Geometry: final body of the model. Coordinates: model frame, mm. A direction names the side the tool comes from. Coordinates: 2 decimals unless noted, no trailing zeros. Write each loop counter-clockwise with the first axis right and the second up, starting at its lowest first coordinate (ties: lowest second). Pieces come first, ordered by that corner, then holes. Notation, with made-up numbers: (-24, 31) - (-18, 31) arc R27 cw to (-18, 52) - close; hole circle Ø4 at (71, 57). An arc over 180 degrees is marked (long way). Put each result on its own line as item: value.
```python
from build123d import *

# Parameters (mm, degrees)
SKETCH1_W           = 57.15
SKETCH1_H           = 50.8
BOSS_EXTRUDE1_DEPTH = 63.5
SKETCH2_R           = 9.506140486
CUT_EXTRUDE1_DEPTH  = 6.35
FILLET1_R           = 7.874
SKETCH3_W           = 47.524607072
SKETCH3_H           = 34.745914464
CUT_EXTRUDE2_DEPTH  = 57.15
FILLET2_R           = 3.81
SKETCH4_R           = 4.44219446
CUT_EXTRUDE3_DEPTH  = 5.08
CUT_EXTRUDE4_DEPTH  = 25.4


with BuildPart() as part:
    # Sketch1 → Boss-Extrude1 (new body)
    with BuildSketch(Plane.XY):
        with Locations((28.575, 25.4)):
            Rectangle(SKETCH1_W, SKETCH1_H)
    extrude(amount=BOSS_EXTRUDE1_DEPTH)

    # Sketch2 → Cut-Extrude1 (cut)
    with BuildSketch(Plane.XY.offset(63.5)):
        with Locations((25.4, 20.32)):
            Circle(SKETCH2_R)
    extrude(amount=-CUT_EXTRUDE1_DEPTH, mode=Mode.SUBTRACT)

    # Fillet1
    fillet1_edges = [part.edges().sort_by_distance(p)[0] for p in [
        (28.575, 50.8, 63.5),
    ]]
    fillet(fillet1_edges, radius=FILLET1_R)

    # Sketch3 → Cut-Extrude2 (cut)
    with BuildSketch(Plane(origin=(57.15, 0, 0), x_dir=(0, 0, -1), z_dir=(1, 0, 0))):
        with Locations((-23.762303536, 17.372957232)):
            Rectangle(SKETCH3_W, SKETCH3_H)
    extrude(amount=-CUT_EXTRUDE2_DEPTH, mode=Mode.SUBTRACT)

    # Fillet2
    fillet2_edges = [part.edges().sort_by_distance(p)[0] for p in [
        (28.575, 34.745914464, 47.524607072),
    ]]
    fillet(fillet2_edges, radius=FILLET2_R)

    # Sketch4 → Cut-Extrude3 (cut)
    with BuildSketch(Plane(origin=(57.15, 0, 0), x_dir=(0, 0, -1), z_dir=(1, 0, 0))):
        with Locations((-55.906607072, 43.18)):
            Circle(SKETCH4_R)
    extrude(amount=-CUT_EXTRUDE3_DEPTH, mode=Mode.SUBTRACT)

    # Sketch5 → Cut-Extrude4 (cut)
    with BuildSketch(Plane(origin=(0, 50.8, 0), x_dir=(1, 0, 0), z_dir=(0, 1, 0))):
        with BuildLine():
            Line((14.081947764, 0), (43.068052236, 0))
            ThreePointArc((43.068052236, 0), (28.575, -14.493052236), (14.081947764, 0))
        make_face()
    extrude(amount=-CUT_EXTRUDE4_DEPTH, mode=Mode.SUBTRACT)


solid = part.part
```
1. Section query A-A (y = 20.32). Return loops of the section in (x, z), then the cut area to 3 significant figures.
Answer below:
outline: (0, 47.52) - (57.15, 47.52) - (57.15, 63.5) - (34.91, 63.5) - (34.91, 57.15) - (15.89, 57.15) - (15.89, 63.5) - (0, 63.5) - close
area: 792 mm²
2. Ray query, probe 1 along Z at (x, y) = (53, 43); probe 2 along Z at (x, y) = (35.5, 8); probe 3 along Y at (x, z) = (25.4, 59.5). Return the intervals inside material, ascending. Write a range as from..to.
Answer below:
probe 1: z = 0..51.47, 60.35..63.5
probe 2: z = 47.52..63.5
probe 3: y = 0..10.81, 29.83..49.78
3. Set-up query: faces 5 (the flat face through (28, 50.8, 27)), 6 (the flat face through (52.07, 43, 56)), 7 (the flat face through (29, 34.746, 27)). Return all of +Z, -Z, +X, -X, +Y, -Y with unobstructed straight access to the full face (end or side cutting, diameter ignored); none if empty.
Answer below:
face 5: +Z, -Z, +X, -X, +Y
face 6: +X
face 7: -Z, +X, -X, -Y
4. Section query D-D (z = 27). Return loops of the section in (x, y), then the cut area to 3 significant figures.
Answer below:
outline: (0, 34.75) - (57.15, 34.75) - (57.15, 50.8) - (0, 50.8) - close
area: 917 mm²
5. Section query C-C (z = 59). Return loops of the section in (x, y), then the cut area to 3 significant figures.
Answer below:
outline: (0, 0) - (57.15, 0) - (57.15, 39.99) - (52.07, 39.99) - (52.07, 46.37) - (57.15, 46.37) - (57.15, 50.04) - (0, 50.04) - close; hole circle Ø19.01 at (25.4, 20.32)
area: 2,540 mm²
6. Pin query (flat end, axial travel): pin 1 Ø2 at (x, y) = (34, 45.5) entering from +Z; pin 2 Ø4 at (x, y) = (11, 17.5) entering from -Z; pin 3 Ø24.5 at (x, y) = (25.4, 20.32) entering from -Z. Return the tip coordinate at first contact, or that it passes through.
Answer below:
pin 1: stops at z = 63.34
pin 2: stops at z = 47.52
pin 3: stops at z = 47.16
7. Mould query, pull axis X, two halves, no side actions, for faces 1 (the cylindrical face through (17.856, 14.536, 60.369)), 2 (the flat face through (7, 43, 0)), 3 (the flat face through (0, 36, 38)), 4 (the flat face through (25, 20, 57.15)). Classes: +X half, -X half, draft (parallel to the pull), parting line (faces both ways), or undercut.
Answer below:
face 1: undercut
face 2: draft
face 3: -X half
face 4: undercut
8. Section query B-B (x = 30). Return loops of the section in (y, z).
Answer below:
outline: (0, 47.52) - (30.94, 47.52) arc R3.81 cw to (34.75, 43.71) - (34.75, 14.42) - (50.8, 14.42) - (50.8, 55.63) arc R7.87 ccw to (42.93, 63.5) - (28.64, 63.5) - (28.64, 57.15) - (12, 57.15) - (12, 63.5) - (0, 63.5) - close
